Autodesk Fusion 360 part; units mm, degrees
sketch "Sketch1" plane through (0, 0, 0) normal (0, 1, 0) x (1, 0, 0)
  line L0 (-100, 12.5) -> (-2, 12.5)
  line L1 (-2, 12.5) -> (0, 14.5)
  line L2 (0, 14.5) -> (0, 18)
  line L3 (0, 18) -> (-2, 20)
  line L4 (-2, 20) -> (-88, 20)
  line L5 (-88, 20) -> (-88, 23)
  line L6 (-88, 23) -> (-90, 25)
  line L7 (-90, 25) -> (-100, 25)
  line L8 (-100, 25) -> (-100, 12.5)
  line L9 (0, 0) -> (-74, 0) construction
  line L10 (-74, -6) -> (-24, -6)
  line L11 (-74, 6) -> (-24, 6)
  arc A0 (-74, 6) -> (-74, -6) centre (-74, 0) ccw
  arc A1 (-24, -6) -> (-24, 6) centre (-24, 0) ccw
  dimension "d1" = 88
  dimension "d2" = 100
  dimension "d3" = 135
  dimension "d4" = 25
  dimension "d5" = 20
  dimension "d6" = 100
  dimension "d7" = 14.5
  dimension "d8" = 135
  dimension "d9" = 45
  dimension "d10" = 2
  dimension "d11" = 2
  dimension "d12" = 90
  dimension "d13" = 12
  dimension "d15" = 12
  dimension "d16" = 24
  dimension "d17" = 74
revolve "Revolve1" add sketch "Sketch1" angle 360 about axis through (1.75, 0, 0) along (1, 0, 0) contours L0 L1 L2 L3 L4 L5 L6 L7 L8
extrude "Extrude1" cut sketch "Sketch1" against normal through all contours L10 L11 A0 A1
equation "d3 = 180 deg - 45 deg"
equation "d4 = ( 50 / 2 ) * 1 mm"
equation "d5 = ( 40 / 2 ) * 1 mm"
equation "d6 = d2"
equation "d7 = ( 29 / 2 ) * 1 mm"
equation "d12 = d1 + 2 mm"
equation "d17 = d16 + 50 mm"
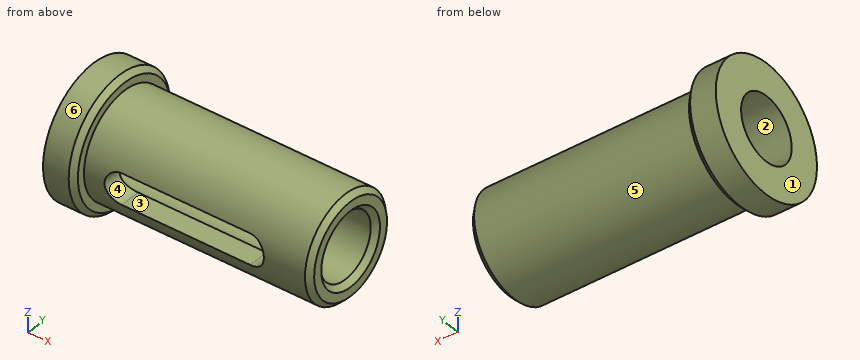
Here's how the part is built. I have some questions about the finished solid (model axes, mm). Face numbers are marked on the shaded views. A direction names the side the tool comes from. Give positions to 0.01 mm unless a question says otherwise; leave off trailing zeros. Order: outer loops, then holes, each group sorted by start corner. A loop starts at its lowest first (then second) coordinate and runs counter-clockwise, first axis right, second up. Notation, with made-up numbers: (-16, -38.75) -> (-2, -38.75) arc R19 cw to (-2, -8.75) -> close; hole circle Ø1 at (71.5, 83.25). An arc over 180 degrees is marked (long way). One line per item, written item: value. Start each with the question number.
1. Will these pins go through, and if not, where does the flat tip stop? pin 1 Ø6.5 at (x, y) = (-45.5, -13) entering from -Z; pin 2 Ø5 at (x, z) = (-59, 18.5) entering from +Y; pin 3 Ø4 at (x, z) = (-79, 0.5) entering from +Y.
2. Imagine slicing it at C-C, the plane x = -14. List the corners of the cut face in (y, z) for me.
3. Imagine slicing it at B-B, the plane z = 0. List the corners of the cut face in (x, y) for me.
4. I need wall thicknesses on probe 1 along Y at (x, z) = (-26, 0); probe 2 along Z at (x, y) = (-5.5, -11); probe 3 along Z at (x, y) = (-19, -0.5). Which ranges of each line are inside material? Lowest first, please. Write a range as from..to.
5. We'd pull the mould along X, two halves only. Please class the marked faces 1, 2 and 3: released by +X, released by -X, zero draft, split by the parting line, or undercut.
6. Imagine slicing it at A-A, the plane y = 0. List the corners of the cut face in (x, z) for me.
7. For the marked faces 4, 5 and 6, which set-ups out of +Z, -Z, +X, -X, +Y, -Y let a thin tool reach every point of the face, with its end or its side?
8. Imagine slicing it at D-D, the plane x = -38. List the corners of the cut face in (y, z) for me, plus the area to 3 significant figures.
Values follow:
1. pin 1: stops at z = -17.46
1. pin 2: stops at y = 12
1. pin 3: stops at y = 20
2. outline: circle Ø40 at (0, 0); hole circle Ø25 at (0, 0)
3. outline: (-100, -25) -> (-90, -25) -> (-88, -23) -> (-88, -20) -> (-80, -20) -> (-80, -12.5) -> (-100, -12.5) -> close; (-100, 12.5) -> (-2, 12.5) -> (0, 14.5) -> (0, 18) -> (-2, 20) -> (-88, 20) -> (-88, 23) -> (-90, 25) -> (-100, 25) -> close; (-18, -20) -> (-2, -20) -> (0, -18) -> (0, -14.5) -> (-2, -12.5) -> (-18, -12.5) -> close
4. probe 1: y = 12.5..20
4. probe 2: z = -16.7..-5.94, 5.94..16.7
4. probe 3: z = -19.99..-12.49, 12.49..19.99
5. face 1: released by -X
5. face 2: zero draft
5. face 3: undercut
6. outline: (-100, -25) -> (-90, -25) -> (-88, -23) -> (-88, -20) -> (-2, -20) -> (0, -18) -> (0, -14.5) -> (-2, -12.5) -> (-100, -12.5) -> close; (-100, 12.5) -> (-2, 12.5) -> (0, 14.5) -> (0, 18) -> (-2, 20) -> (-88, 20) -> (-88, 23) -> (-90, 25) -> (-100, 25) -> close
7. face 4: -Y
7. face 5: +X
7. face 6: +X, -X
8. outline: (-19.08, -6) arc R20 ccw (long way) to (-19.08, 6) -> (-10.97, 6) arc R12.5 cw (long way) to (-10.97, -6) -> close
8. area: 673 mm2
